Read the model definition and answer for the solid it produces. Units are mm, in the model's axes. Face numbers are marked on the shaded views. Round coordinates to 2 decimals unless told otherwise and drop trailing zeros. Loops run counter-clockwise (first coordinate to the right, second up) from the corner with the lowest first, then second, coordinate; pieces in that order, holes last. Notation, with made-up numbers: M 18,63 L 27,63 A18 ccw 27,96 Z; hole C 69.5,24 d1. An arc over 180 degrees is marked long. Write each question's results on one line, items separated by ' | '.
from build123d import *

# Parameters (mm, degrees)
F0_R     = 317.5
F0_R_2   = 266.7
F1_DEPTH = 6.35
F2_R     = 308.61
F2_R_2   = 301.625
F3_DEPTH = 50.8
F2_R_3   = 313.382665
F4_DEPTH = 19.05
F5_SIZE  = 2.54


with BuildPart() as f1:
    # F0 (on Top) → F1 (new body)
    with BuildSketch(Plane.XY):
        Circle(F0_R)
        Circle(F0_R_2, mode=Mode.SUBTRACT)
    extrude(amount=F1_DEPTH)

    # F2 (on face) → F3 (join)
    with BuildSketch(Plane(origin=(0, 0, 0), x_dir=(1, 0, 0), z_dir=(0, 0, -1))):
        Circle(F2_R)
        Circle(F2_R_2, mode=Mode.SUBTRACT)
    extrude(amount=F3_DEPTH)

    # F2 (on face) → F4 (join)
    with BuildSketch(Plane(origin=(0, 0, 0), x_dir=(1, 0, 0), z_dir=(0, 0, -1))):
        Circle(F2_R_3)
        Circle(F2_R, mode=Mode.SUBTRACT)
    extrude(amount=F4_DEPTH)

    # F5
    f5_edges = [f1.edges().sort_by_distance(p)[0] for p in [
        (-313.382665, 0, -19.05),
        (-317.5, 0, 0),
        (-308.61, 0, -50.8),
    ]]
    chamfer(f5_edges, length=F5_SIZE)


solid = f1.part
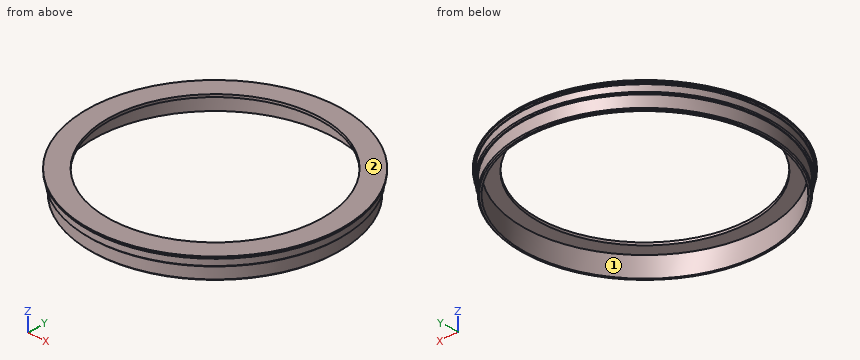
Item 1: The mould has two halves that part along X. Classify the marked faces 1 and 2: pulls with the +X half, pulls with the -X half, needs draft (parallel to the pull), parting line crosses it, or undercut.
Outcome:
face 1: undercut | face 2: needs draft
Item 2: Straight lines are drawn through the part: line 1 (X direction, y = 0, z = -26) (3 decimals); line 2 (Y direction, x = 0, z = 4). For each, find the intervals that lie inside material, in ascending order.
Outcome:
line 1: x = -308.61 to -301.625, 301.625 to 308.61 | line 2: y = -317.5 to -266.7, 266.7 to 317.5
Item 3: The part is cut by section C-C (z = -34.5). Determine the outline of the cut face in (x, y) (3 decimals).
Outcome:
outline: C 0,0 d617.22; hole C 0,0 d603.25
Item 4: Flat-ended cylindrical pins translate along their axes: pin 1 (4 mm diameter, centred on y = 87, z = -38, fed in from -X); pin 2 (1.5 mm diameter, centred on y = 49.5, z = -13.5, fed in from +X); pin 3 (1.5 mm diameter, centred on y = 69.5, z = -17, fed in from +X). Find the tip coordinate at first contact, or state that the pin passes through.
Outcome:
pin 1: stops at x = -296.67 | pin 2: stops at x = 309.57 | pin 3: stops at x = 305.71
Item 5: The part is cut by section A-A (x = 0). Determine the outline of the cut face in (y, z) (3 decimals), plus the area to 3 significant figures.
Outcome:
outline: M -317.5,2.54 L -314.96,0 L -313.383,0 L -313.383,-16.51 L -310.843,-19.05 L -308.61,-19.05 L -308.61,-48.26 L -306.07,-50.8 L -301.625,-50.8 L -301.625,0 L -266.7,0 L -266.7,6.35 L -317.5,6.35 Z; M 266.7,0 L 301.625,0 L 301.625,-50.8 L 306.07,-50.8 L 308.61,-48.26 L 308.61,-19.05 L 310.843,-19.05 L 313.383,-16.51 L 313.383,0 L 314.96,0 L 317.5,2.54 L 317.5,6.35 L 266.7,6.35 Z | area: 1,520 mm2
